Autodesk Inventor part; units mm, degrees
ref_plane "YZ Plane" through (0, 0, 0) normal (1, 0, 0) x (0, 1, 0)
ref_plane "XZ Plane" through (0, 0, 0) normal (0, 1, 0) x (-1, 0, 0)
ref_plane "XY Plane" through (0, 0, 0) normal (0, 0, 1) x (1, 0, 0)
sketch "Sketch1" plane through (0, 0, 0) normal (0, 0, 1) x (1, 0, 0)
  line L0 (0, 0) -> (15, 0)
  line L1 (0, 0) -> (-15, 0)
  line L2 (0, 0) -> (5, 0)
  circle A0 centre (-15, 0) radius 1.25
  circle A1 centre (15, 0) radius 1.25
  circle A2 centre (-15, 0) radius 2
  circle A3 centre (15, 0) radius 2
  line L3 (-15, 2) -> (15, 2)
  line L4 (-15, -2) -> (15, -2)
  line L5 (-15, 2) -> (-9, 2)
  line L6 (-9, 2) -> (-9, -2)
  line L7 (-9, -2) -> (-15, -2)
  line L8 (-15, -2) -> (-15, 2)
  line L9 (15, 2) -> (12.5, 2)
  line L10 (15, -2) -> (15, 2)
  arc A4 (-9, -2) -> (-9, 2) centre (-11.2361, 0) ccw
  line L11 (5, 0) -> (1, 0)
  line L12 (5, 2) -> (5, 2)
  line L13 (5, 0) -> (9, 0)
  line L14 (-15, 2) -> (-14.5, 2)
  line L15 (-15, -2) -> (-14.5, -2)
  arc A5 (-14.5, -2) -> (-14.5, 2) centre (-14.5, 0) ccw
  line L16 (15, 0) -> (7, 0)
  line L17 (15, 2) -> (5, 2)
  line L18 (15, -2) -> (5, -2)
  arc A6 (5, -2) -> (5, 2) centre (5, 0) ccw
  point P0 (-9, 2)
  dimension "d1" = 15
  dimension "d2" = 15
  dimension "d4" = 2.5
  dimension "d6" = 2.5
  dimension "d7" = 4
  dimension "d8" = 4
  dimension "d10" = 6
  dimension "d16" = 4
  dimension "d17" = 3
  dimension "d24" = 0.5
  dimension "d25" = 0.5
  dimension "d26" = 2
  dimension "d37" = 8
  dimension "d38" = 10
  dimension "d45" = 10
extrude "Extrusion6" add sketch "Sketch1" along normal mid plane 2 contours A4 L6 L1 | L1 L6 A4 | L6 L4 A5 L1 | L1 A5 L3 L6 | A6 L3 A3 L0 | L0 A3 L4 A6 | A5 L4 A2 L1 | L1 A2 L3 A5 | A2 L8 A0 L1 | L1 A0 L8 A2 | A2 L8 A0 | L10 A1 A3 | A3 L0 A1 L10 | A3 L10 A1 L0
extrude "Extrusion7" add sketch "Sketch1" along normal mid plane 4 contours L1 A4 L3 A6 L0 | L0 A6 L4 A4 L1
move or copy body "Move Body1" bodies to move or copy 1 copy no rotation origin (0, 0, 0) rotation axis (0, 0, 1) rotation angle 180
properties part number "link7" material "Aluminum 6061"
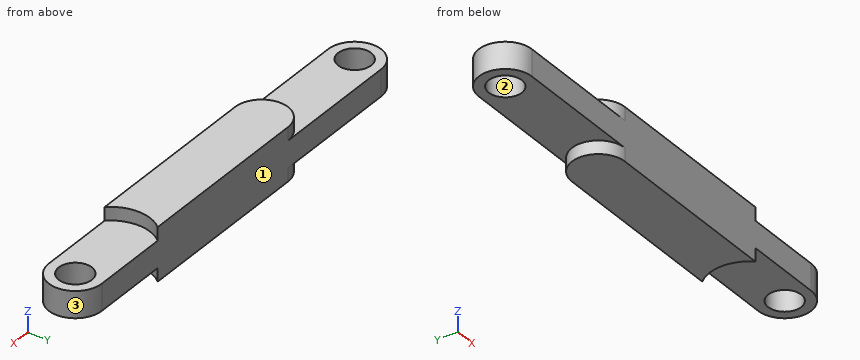
For this review, take the finished solid that the model builds, in its own axes (mm). Face numbers are marked on the shaded views. Coordinates: 2 decimals unless noted, no trailing zeros. Write each loop counter-clockwise with the first axis right and the second up, starting at its lowest first coordinate (ties: lowest second). Pieces come first, ordered by that corner, then holes.
(1) Add section A-A on y = -0.6. Give the boundary of the cut face in (x, z), then the cut area to 3 significant figures.
(2) Add section C-C on z = -0.05. Give the boundary of the cut face in (x, y), then the cut area to 3 significant figures.
(3) Add section D-D on z = 1.3. Give the boundary of the cut face in (x, y).
(4) Wall thickness on probe 1 along X at (y, z) = (0, 0.1); probe 2 along Y at (x, z) = (-15, 0.5); probe 3 along X at (y, z) = (1.1, 0.7): over which ranges is each line inside the solid? List them lowest first.
(5) For pin 1 Ø1 at (x, y) = (11.5, -0.5) entering from -Z; pin 2 Ø1.2 at (x, y) = (-11.5, 0.5) entering from +Z, all flat-tipped, find the tip position at first contact; note any pin that passes through.
(6) The part is to be moulded in two halves that separate along Y. For the marked faces 1, 2 and 3, say which applies: +Y half, -Y half, draft (parallel to the pull), parting line (faces both ways), or undercut.
(7) Add section B-B on x = -6. Give the boundary of the cut face in (y, z), then the cut area to 3 significant figures.
Answer sheet:
1. outline: (-16.91, -1) - (-16.1, -1) - (-16.1, 1) - (-16.91, 1) - close; (-13.9, -1) - (-6.91, -1) - (-6.91, -2) - (8.3, -2) - (8.3, -1) - (13.9, -1) - (13.9, 1) - (8.3, 1) - (8.3, 2) - (-6.91, 2) - (-6.91, 1) - (-13.9, 1) - close; (16.1, -1) - (16.91, -1) - (16.91, 1) - (16.1, 1) - close
1. area: 89.3 mm2
2. outline: (-15, -2) - (15, -2) arc R2 ccw to (15, 2) - (-15, 2) arc R2 ccw to start; hole circle Ø2.5 at (-15, 0); hole circle Ø2.5 at (15, 0)
2. area: 123 mm2
3. outline: (-5, -2) - (9, -2) arc R3 cw to (9, 2) - (-5, 2) arc R2 ccw to start
4. probe 1: x = -17 to -16.25, -13.75 to 13.75, 16.25 to 17
4. probe 2: y = -2 to -1.25, 1.25 to 2
4. probe 3: x = -16.67 to -15.59, -14.41 to 14.41, 15.59 to 16.67
5. pin 1: stops at z = -1
5. pin 2: stops at z = 1
6. face 1: +Y half
6. face 2: undercut
6. face 3: parting line
7. outline: (-2, -1) - (-1.73, -1) - (-1.73, -2) - (1.73, -2) - (1.73, -1) - (2, -1) - (2, 1) - (1.73, 1) - (1.73, 2) - (-1.73, 2) - (-1.73, 1) - (-2, 1) - close
7. area: 14.9 mm2
